Design review of the part built by this model. Coordinates are the model's own, in mm. A direction names the side the tool comes from. Round coordinates to 2 decimals unless told otherwise and drop trailing zeros. Order: outer loops, then holes, each group sorted by start corner. A loop starts at its lowest first (then second) coordinate and runs counter-clockwise, first axis right, second up. Notation, with made-up numbers: M 85.5,17.5 L 95.5,17.5 A22 cw 95.5,36.5 Z; hole C 5.5,33 d5. An arc over 180 degrees is marked long. Use a Markdown table: item, result. Add a question column.
(1) For pin 1 (12 mm diameter, centred on y = 63, z = -14.5, fed in from -X); pin 2 (1 mm diameter, centred on y = 51.5, z = 4.5, fed in from -X); pin 3 (6 mm diameter, centred on y = 50, z = 17.5, fed in from +X), all flat-tipped, find the tip position at first contact; note any pin that passes through.
(2) To check wall thickness, follow probe 1 along Y at (x, z) = (-22, 4); probe 2 along X at (y, z) = (79, -1); probe 3 along X at (y, z) = (71, 13.5). State the ranges of each line that lie inside material, in increasing order. Write a range as from..to.
(3) Take a section at D-D (y = 17). Write out the cut boundary in (x, z), then the cut area to 3 significant figures.
(4) Take a section at C-C (y = 69). Write out the cut boundary in (x, z).
(5) Machinability: for faces 1 (the face through (10.382, 59.44, -19.961)), 2 (the face through (0, 0, 0)), which of the approach directions +Z, -Z, +X, -X, +Y, -Y give a long, thin tool a straight path to every point of the face, cutting with its end or side? Answer none if there is none.
(6) Take a section at B-B (z = 0). Write out the cut boundary in (x, y), then the cut area to 3 significant figures.
(7) Take a section at A-A (x = 0). Write out the cut boundary in (y, z), then the cut area to 3 significant figures.
```python
from build123d import *

# Parameters (mm, degrees)
F0_R     = 22.5
F0_R_2   = 30
F1_DEPTH = 20
F2_DEPTH = 100
F3_SIZE  = 5
F4_R     = 8


with BuildPart() as f1:
    # F0 (on Front) → F1 (new body)
    with BuildSketch(Plane.XZ):
        Circle(F0_R)
        Circle(F0_R_2)
        Circle(F0_R, mode=Mode.SUBTRACT)
    extrude(amount=-F1_DEPTH)

    # F0 (on Front) → F2 (join)
    with BuildSketch(Plane.XZ):
        Circle(F0_R)
    extrude(amount=-F2_DEPTH)

    # F3
    f3_edges = [f1.edges().sort_by_distance(p)[0] for p in [
        (-30, 20, 0),
    ]]
    chamfer(f3_edges, length=F3_SIZE)

    # F4
    f4_edges = [f1.edges().sort_by_distance(p)[0] for p in [
        (-30, 0, 0),
    ]]
    fillet(f4_edges, radius=F4_R)


solid = f1.part
```
Verdict:
| question | item | result |
|---|---|---|
| 1 | pin 1 | stops at x = -20.83 |
| 1 | pin 2 | stops at x = -22.14 |
| 1 | pin 3 | stops at x = 17.2 |
| 2 | probe 1 | y = 0.01..100 |
| 2 | probe 2 | x = -22.48..22.48 |
| 2 | probe 3 | x = -18..18 |
| 3 | outline | C 0,0 d56 |
| 3 | area | 2,460 mm^2 |
| 4 | outline | C 0,0 d45 |
| 5 | face 1 | +Y |
| 5 | face 2 | +Z, -Z, +X, -X, -Y |
| 6 | outline | M -30,8 A8 ccw -22,0 L 22,0 A8 ccw 30,8 L 30,15 L 25,20 L 22.5,20 L 22.5,100 L -22.5,100 L -22.5,20 L -25,20 L -30,15 Z |
| 6 | area | 4,750 mm^2 |
| 7 | outline | M 0,-22 A8 ccw 8,-30 L 15,-30 L 20,-25 L 20,-22.5 L 100,-22.5 L 100,22.5 L 20,22.5 L 20,25 L 15,30 L 8,30 A8 ccw 0,22 Z |
| 7 | area | 4,750 mm^2 |
